```python
from build123d import *

# Parameters (mm, degrees)
BOSS_EXTRUDE6_DEPTH              = 53.34
BOSS_EXTRUDE6_DEPTH_BACK         = 101.6
CUT_EXTRUDE8_REACH               = 902.262
CUT_EXTRUDE8_DIRECTION_2_REACH   = 902.262
SKETCH15_R                       = 19.05
BOSS_EXTRUDE8_DEPTH              = 127
CUT_EXTRUDE9_REACH               = 1709.816
SKETCH16_W                       = 38.1
SKETCH16_H                       = 10.414
CUT_EXTRUDE9_DIRECTION_2_REACH   = 1709.816
SKETCH17_R                       = 15.24
BOSS_EXTRUDE9_DEPTH              = 127
BOSS_EXTRUDE9_DIRECTION_2_REACH  = 1707.258
SKETCH18_R                       = 15.24
BOSS_EXTRUDE10_DEPTH             = 127
BOSS_EXTRUDE10_DIRECTION_2_REACH = 1704.799
CUT_EXTRUDE10_REACH              = 1704.799
CUT_EXTRUDE10_DIRECTION_2_REACH  = 1704.799


with BuildPart() as part:
    # Sketch12 → Boss-Extrude6 (new, two sides: drawn at the far end of the back side and taken through both)
    with BuildSketch(Plane.XY.offset(-BOSS_EXTRUDE6_DEPTH_BACK)):
        Polygon((-203.2, 241.3), (203.2, 241.3), (787.471663752, -383.669201703), (787.471663752, -424.309201703), (762.071663752, -424.309201703), (762.071663752, -386.209201703), (203.2, 215.9), (-203.2, 215.9), (-762.071663752, -386.209201703), (-762.071663752, -424.309201703), (-787.471663752, -424.309201703), (-787.471663752, -383.669201703), align=None)
    extrude(amount=BOSS_EXTRUDE6_DEPTH + BOSS_EXTRUDE6_DEPTH_BACK)

    # Cut-Extrude8: up to this plane
    cut_extrude8_end = Plane(origin=(-203.2, 241.3, -101.6), z_dir=(-0.7304911811601322, 0.6829221289775833, 0))
    # Sketch14 → Cut-Extrude8 (cut, up to the surface)
    with BuildSketch(Plane(origin=(0, 0, 0), x_dir=(0, 0, -1), z_dir=(1, 0, 0)), mode=Mode.PRIVATE) as cut_extrude8_sk1:
        Polygon((0, 241.3), (0, 215.9), (-53.34, -386.209201703), (-53.34, 241.3), align=None)
    cut_extrude8_tool1 = split(extrude(cut_extrude8_sk1.sketch, amount=-CUT_EXTRUDE8_REACH, mode=Mode.PRIVATE), bisect_by=cut_extrude8_end, keep=Keep.BOTH, mode=Mode.PRIVATE)
    add(cut_extrude8_tool1.solids().sort_by_distance((0, 31.800889, 34.868308))[0], mode=Mode.SUBTRACT)
    # Sketch14 → Cut-Extrude8 (cut, up to the surface)
    with BuildSketch(Plane(origin=(0, 0, 0), x_dir=(0, 0, -1), z_dir=(1, 0, 0)), mode=Mode.PRIVATE) as cut_extrude8_sk2:
        Polygon((101.6, 215.9), (-15.24, -386.209201703), (-15.24, -424.309201703), (101.6, -424.309201703), align=None)
    cut_extrude8_tool2 = split(extrude(cut_extrude8_sk2.sketch, amount=-CUT_EXTRUDE8_REACH, mode=Mode.PRIVATE), bisect_by=cut_extrude8_end, keep=Keep.BOTH, mode=Mode.PRIVATE)
    add(cut_extrude8_tool2.solids().sort_by_distance((0, -210.192787, -60.465735))[0], mode=Mode.SUBTRACT)

    # Cut-Extrude8 direction 2: up to this plane
    cut_extrude8_direction_2_end = Plane(origin=(203.2, 241.3, -101.6), z_dir=(0.7304911811601321, 0.6829221289775835, 0))
    # Sketch14 → Cut-Extrude8 direction 2 (cut, up to the surface)
    with BuildSketch(Plane(origin=(0, 0, 0), x_dir=(0, 0, -1), z_dir=(1, 0, 0)), mode=Mode.PRIVATE) as cut_extrude8_direction_2_sk1:
        Polygon((0, 241.3), (0, 215.9), (-53.34, -386.209201703), (-53.34, 241.3), align=None)
    cut_extrude8_direction_2_tool1 = split(extrude(cut_extrude8_direction_2_sk1.sketch, amount=CUT_EXTRUDE8_DIRECTION_2_REACH, mode=Mode.PRIVATE), bisect_by=cut_extrude8_direction_2_end, keep=Keep.BOTH, mode=Mode.PRIVATE)
    add(cut_extrude8_direction_2_tool1.solids().sort_by_distance((0, 31.800889, 34.868308))[0], mode=Mode.SUBTRACT)
    # Sketch14 → Cut-Extrude8 direction 2 (cut, up to the surface)
    with BuildSketch(Plane(origin=(0, 0, 0), x_dir=(0, 0, -1), z_dir=(1, 0, 0)), mode=Mode.PRIVATE) as cut_extrude8_direction_2_sk2:
        Polygon((101.6, 215.9), (-15.24, -386.209201703), (-15.24, -424.309201703), (101.6, -424.309201703), align=None)
    cut_extrude8_direction_2_tool2 = split(extrude(cut_extrude8_direction_2_sk2.sketch, amount=CUT_EXTRUDE8_DIRECTION_2_REACH, mode=Mode.PRIVATE), bisect_by=cut_extrude8_direction_2_end, keep=Keep.BOTH, mode=Mode.PRIVATE)
    add(cut_extrude8_direction_2_tool2.solids().sort_by_distance((0, -210.192787, -60.465735))[0], mode=Mode.SUBTRACT)

    # Sketch15 → Boss-Extrude8 (add)
    with BuildSketch(Plane.ZY.offset(762.071663752)):
        with Locations((34.29, -394.845201703)):
            Circle(SKETCH15_R)
    boss_extrude8 = extrude(amount=BOSS_EXTRUDE8_DEPTH)

    # Mirror2: Boss-Extrude8 across plane
    add(boss_extrude8.mirror(Plane(origin=(0, 0, 0), x_dir=(0, 0, 1), z_dir=(1, 0, 0))))

    # Cut-Extrude9: up to this face of the body (flat: up to its plane)
    cut_extrude9_end = Plane(part.part.faces().sort_by_distance((-787.471663752, -416.434815963, 34.29))[0])
    # Sketch16 → Cut-Extrude9 (cut, up to the picked face)
    with BuildSketch(Plane.ZY.offset(762.071663752), mode=Mode.PRIVATE) as cut_extrude9_sk1:
        with Locations((34.29, -419.102201703)):
            Rectangle(SKETCH16_W, SKETCH16_H)
    cut_extrude9_tool1 = split(extrude(cut_extrude9_sk1.sketch, amount=CUT_EXTRUDE9_REACH, mode=Mode.PRIVATE), bisect_by=cut_extrude9_end, keep=Keep.BOTH, mode=Mode.PRIVATE)
    add(cut_extrude9_tool1.solids().sort_by(Axis((-762.071664, -419.102202, 34.29), (-1, 0, 0)))[0], mode=Mode.SUBTRACT)

    # Cut-Extrude9 direction 2: up to this face of the body (flat: up to its plane)
    cut_extrude9_direction_2_end = Plane(part.part.faces().sort_by_distance((787.471663752, -416.434815963, 34.29))[0])
    # Sketch16 → Cut-Extrude9 direction 2 (cut, up to the picked face)
    with BuildSketch(Plane.ZY.offset(762.071663752), mode=Mode.PRIVATE) as cut_extrude9_direction_2_sk1:
        with Locations((34.29, -419.102201703)):
            Rectangle(SKETCH16_W, SKETCH16_H)
    cut_extrude9_direction_2_tool1 = split(extrude(cut_extrude9_direction_2_sk1.sketch, amount=-CUT_EXTRUDE9_DIRECTION_2_REACH, mode=Mode.PRIVATE), bisect_by=cut_extrude9_direction_2_end, keep=Keep.BOTH, mode=Mode.PRIVATE)
    add(cut_extrude9_direction_2_tool1.solids().sort_by(Axis((-762.071664, -419.102202, 34.29), (1, 0, 0)))[0], mode=Mode.SUBTRACT)

    # Sketch17 → Boss-Extrude9 (add)
    with BuildSketch(Plane.ZY.offset(762.071663752)):
        with Locations((34.29, -342.521201703)):
            Circle(SKETCH17_R)
    extrude(amount=BOSS_EXTRUDE9_DEPTH)

    # Boss-Extrude9 direction 2: up to this face of the body (flat: up to its plane)
    boss_extrude9_direction_2_end = Plane(part.part.faces().sort_by_distance((-449.243763763, -21.881982223, -17.095411005))[0])
    # Sketch17 → Boss-Extrude9 direction 2 (add, up to the picked face)
    with BuildSketch(Plane.ZY.offset(762.071663752), mode=Mode.PRIVATE) as boss_extrude9_direction_2_sk1:
        with Locations((34.29, -342.521201703)):
            Circle(SKETCH17_R)
    boss_extrude9_direction_2_tool1 = split(extrude(boss_extrude9_direction_2_sk1.sketch, amount=-BOSS_EXTRUDE9_DIRECTION_2_REACH, mode=Mode.PRIVATE), bisect_by=boss_extrude9_direction_2_end, keep=Keep.BOTH, mode=Mode.PRIVATE)
    add(boss_extrude9_direction_2_tool1.solids().sort_by(Axis((-762.071664, -342.521202, 34.29), (1, 0, 0)))[0])

    # Sketch18 → Boss-Extrude10 (add)
    with BuildSketch(Plane.ZY.offset(-759.531663752)):
        with Locations(Location((34.117724321, -342.561697921, 0), (0, 0, 270))):
            Circle(SKETCH18_R)
    extrude(amount=-BOSS_EXTRUDE10_DEPTH)

    # Boss-Extrude10 direction 2: up to this face of the body (flat: up to its plane)
    boss_extrude10_direction_2_end = Plane(part.part.faces().sort_by_distance((449.243763763, -21.881982223, -17.095411005))[0])
    # Sketch18 → Boss-Extrude10 direction 2 (add, up to the picked face)
    with BuildSketch(Plane.ZY.offset(-759.531663752), mode=Mode.PRIVATE) as boss_extrude10_direction_2_sk1:
        with Locations(Location((34.117724321, -342.561697921, 0), (0, 0, 270))):
            Circle(SKETCH18_R)
    boss_extrude10_direction_2_tool1 = split(extrude(boss_extrude10_direction_2_sk1.sketch, amount=BOSS_EXTRUDE10_DIRECTION_2_REACH, mode=Mode.PRIVATE), bisect_by=boss_extrude10_direction_2_end, keep=Keep.BOTH, mode=Mode.PRIVATE)
    add(boss_extrude10_direction_2_tool1.solids().sort_by(Axis((759.531664, -342.561698, 34.117724), (-1, 0, 0)))[0])

    # Cut-Extrude10: up to this face of the body (flat: up to its plane)
    cut_extrude10_end = Plane(part.part.faces().sort_by_distance((889.071663752, -394.845201703, 34.29))[0])
    # Sketch19 → Cut-Extrude10 (cut, up to the picked face)
    with BuildSketch(Plane.ZY.offset(-759.531663752), mode=Mode.PRIVATE) as cut_extrude10_sk1:
        Polygon((53.34, -413.895201703), (53.34, -360.809201703), (53.34, -357.761201703), (9.719632082, -357.761201703), (9.719632082, -413.895201703), (10.311100074, -413.895201703), align=None)
    cut_extrude10_tool1 = split(extrude(cut_extrude10_sk1.sketch, amount=-CUT_EXTRUDE10_REACH, mode=Mode.PRIVATE), bisect_by=cut_extrude10_end, keep=Keep.BOTH, mode=Mode.PRIVATE)
    add(cut_extrude10_tool1.solids().sort_by(Axis((759.531664, -385.828202, 31.529816), (1, 0, 0)))[0], mode=Mode.SUBTRACT)

    # Cut-Extrude10 direction 2: up to this face of the body (flat: up to its plane)
    cut_extrude10_direction_2_end = Plane(part.part.faces().sort_by_distance((-889.071663752, -394.845201703, 34.29))[0])
    # Sketch19 → Cut-Extrude10 direction 2 (cut, up to the picked face)
    with BuildSketch(Plane.ZY.offset(-759.531663752), mode=Mode.PRIVATE) as cut_extrude10_direction_2_sk1:
        Polygon((53.34, -413.895201703), (53.34, -360.809201703), (53.34, -357.761201703), (9.719632082, -357.761201703), (9.719632082, -413.895201703), (10.311100074, -413.895201703), align=None)
    cut_extrude10_direction_2_tool1 = split(extrude(cut_extrude10_direction_2_sk1.sketch, amount=CUT_EXTRUDE10_DIRECTION_2_REACH, mode=Mode.PRIVATE), bisect_by=cut_extrude10_direction_2_end, keep=Keep.BOTH, mode=Mode.PRIVATE)
    add(cut_extrude10_direction_2_tool1.solids().sort_by(Axis((759.531664, -385.828202, 31.529816), (-1, 0, 0)))[0], mode=Mode.SUBTRACT)


solid = part.part
```
Geometry check sheet. Reference: the model listing, model coordinates, mm. A direction names the side the tool comes from. Give positions to 0.01 mm unless a question says otherwise; leave off trailing zeros. Loops run counter-clockwise (first coordinate to the right, second up) from the corner with the lowest first, then second, coordinate; pieces in that order, holes last. Notation, with made-up numbers: M 23.25,5.5 L 34.25,5.5 A13 ccw 34.25,29.5 Z; hole C 66.25,-36 d4. An arc over 180 degrees is marked long. Write item = value, one per line. Start each with the question number.
1. Go/stop test with flat-tipped pins: P1, Ø12, axis at y = 1.5, z = 8.5, coming from the -X side; P2, Ø6, axis at x = 287, z = -10, coming from the +Y side; P3, Ø7.5, axis at x = -75.5, y = 234, coming from the +Z side. Record where each tip stops, or that it passes through.
2. Tool access check on faces 4 (the face through (-406.54, -3.17, -9.52)), 5 (the face through (-812.72, -327.41, 32.31)), 6 (the face through (811.35, -327.336, 34.772)). Record the directions out of +Z, -Z, +X, -X, +Y, -Y that give a thin tool (end or side, any length) a straight path to the whole face; none if there is none.
3. Draft check along X on faces 1 (the face through (-889.072, -342, 34)), 2 (the face through (502.661, -90.839, 27.174)), 3 (the face through (3, 215.9, -52)). Enter one of: +X half, -X half, draft (parallel to the pull), parting line (faces both ways), or undercut.
4. Section check A-A, the plane y = -266.5. Enter the section's corners in (x, z).
5. Section check D-D, the plane y = -148.5. Enter the section's corners in (x, z), plus the area to 3 significant figures.
6. Section check B-B, the plane z = -48. Enter the section's corners in (x, y), plus the area to 3 significant figures.
7. Section check C-C, the plane x = 93. Enter the section's corners in (y, z).
8. Thickness scan on probe 1 along X at (y, z) = (23, 8); probe 2 along X at (y, z) = (-70, -21.5); probe 3 along Y at (x, z) = (103.5, -94). Record the ranges inside material, lowest first.
Values follow:
q1.P1 = -432.99
q1.P2 = 154.87
q1.P3 = 0
q2.face_4 = +Z, -Z, -Y
q2.face_5 = -X
q2.face_6 = +X
q3.face_1 = -X half
q3.face_2 = draft
q3.face_3 = undercut
q4.outline = M -677.93,-7.99 L -650.96,-7.99 L -650.96,42.74 L -677.93,42.74 Z; M 650.96,-7.99 L 677.93,-7.99 L 677.93,42.74 L 650.96,42.74 Z
q5.outline = M -567.62,-30.89 L -541.43,-30.89 L -541.43,32.28 L -567.62,32.28 Z; M 541.43,-30.89 L 567.62,-30.89 L 567.62,32.28 L 541.43,32.28 Z
q5.area = 3,310 mm^2
q6.outline = M -485.17,-60.32 L -459.58,-60.32 L -203.2,215.9 L 203.2,215.9 L 459.58,-60.32 L 485.17,-60.32 L 203.2,241.3 L -203.2,241.3 Z
q6.area = 24,600 mm^2
q7.outline = M 215.9,-101.6 L 241.3,-101.6 L 241.3,0 L 215.9,0 Z
q8.probe_1 = -407.28 to -382.25, 382.25 to 407.28
q8.probe_2 = -494.23 to -468.57, 468.57 to 494.23
q8.probe_3 = 215.9 to 241.3
